Answer from the drawing. Dimensions are ordinates in mm from the lowest x, y and z of the part. A direction names the side the tool comes from. Round coordinates to 2 decimals unless told otherwise and drop trailing zeros. Loops run counter-clockwise (first coordinate to the right, second up) from the corner with the lowest first, then second, coordinate; pieces in that order, holes last. Notation, with made-up numbers: M 24.5,36.25 L 63.5,36.25 A13 ccw 63.5,59.25 Z; hole C -30.5,26.25 d9. An arc over 180 degrees is marked long. Answer as CSV lines item,"result".
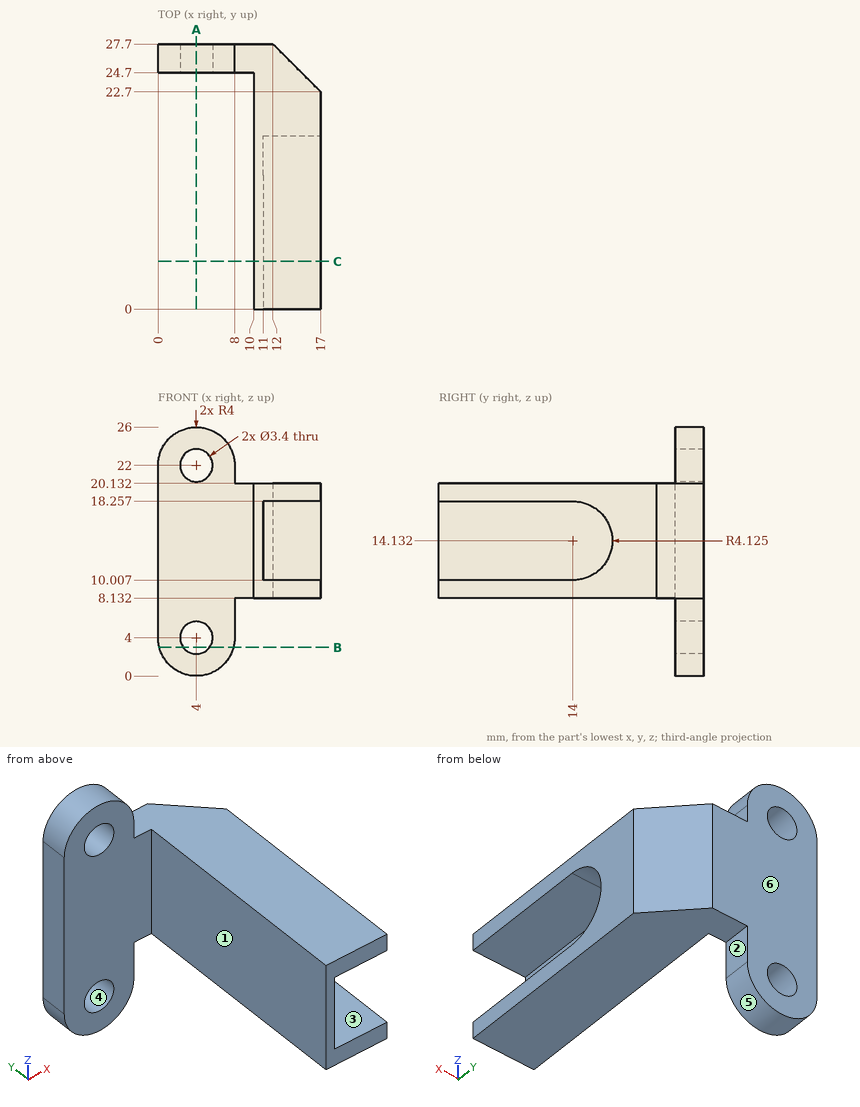
1) A tool of negligible diameter and unlimited length cuts with its end or side. For the marked faces 1, 2 and 3, from which of +Z, -Z, +X, -X, +Y, -Y can it reach the whole face along a straight path? Write none if from no direction.
Evaluation:
face 1,"+Z, -Z, -X, -Y"
face 2,"-Z, +X, +Y, -Y"
face 3,"+X, -Y"
2) Determine the mould class of the marked faces 4, 5 and 6 for opening direction Z: released by +Z, released by -Z, zero draft, split by the parting line, or undercut.
Evaluation:
face 4,"undercut"
face 5,"released by -Z"
face 6,"zero draft"
3) Find section B-B, the plane z = 3. Give the vertices of the cut face in (x, y) (1 decimal), then the cut area to 3 significant figures.
Evaluation:
outline,"M 0.1,24.7 L 2.6,24.7 L 2.6,27.7 L 0.1,27.7 Z; M 5.4,24.7 L 7.9,24.7 L 7.9,27.7 L 5.4,27.7 Z"
area,"15.0 mm^2"
4) Find section C-C, the plane y = 5. Give the vertices of the cut face in (x, z).
Evaluation:
outline,"M 10,8.13 L 17,8.13 L 17,10.01 L 11,10.01 L 11,18.26 L 17,18.26 L 17,20.13 L 10,20.13 Z"
5) Each of these flat-tipped pins is pushed along its axis until it touches: P1, Ø3, axis at y = 15.5, z = 16, coming from the +X side; P2, Ø9.5, axis at y = 10.5, z = 12.5, coming from the -X side; P3, Ø2, axis at x = 14.5, z = 18.5, coming from the +Y side. Where does it stop, or does it pass through?
Evaluation:
P1,"stops at x = 11"
P2,"stops at x = 10"
P3,"stops at y = 26.2"
6) Straight lines are drawn through the part: line 1 (Z direction, x = 4, y = 26.85); line 2 (X direction, y = 25.4, z = 4); line 3 (X direction, y = 21.5, z = 18.5). For each, find the intervals that lie inside material, in ascending order.
Evaluation:
line 1,"z = 0 to 2.3, 5.7 to 20.3, 23.7 to 26"
line 2,"x = 0 to 2.3, 5.7 to 8"
line 3,"x = 10 to 17"
7) Find section A-A, the plane x = 4. Give the vertices of the cut face in (y, z).
Evaluation:
outline,"M 24.7,0 L 27.7,0 L 27.7,2.3 L 24.7,2.3 Z; M 24.7,5.7 L 27.7,5.7 L 27.7,20.3 L 24.7,20.3 Z; M 24.7,23.7 L 27.7,23.7 L 27.7,26 L 24.7,26 Z"
